```python
from build123d import *


with BuildPart() as part:
    # 草图1 → 旋转1 (revolve)
    with BuildSketch(Plane.XY, mode=Mode.PRIVATE) as revolve_1_sk:
        Polygon((10, 0), (0, 0), (0, 3.521877004), (0.272997582, 4), (0.545995165, 3.521877004), (0.818992747, 4), (1.091990329, 3.521877004), (1.364987912, 4), (1.637985494, 3.521877004), (1.910983076, 4), (2.183980659, 3.521877004), (2.456978241, 4), (2.729975823, 3.521877004), (3.002973406, 4), (3.275970988, 3.521877004), (3.548968571, 4), (3.821966153, 3.521877004), (4.094963735, 4), (4.367961318, 3.521877004), (4.6409589, 4), (4.913956482, 3.521877004), (5.186954065, 4), (5.459951647, 3.521877004), (5.732949229, 4), (6.005946812, 3.521877004), (6.278944394, 4), (6.551941976, 3.521877004), (6.824939559, 4), (7.097937141, 3.521877004), (7.236117111, 3.763882889), (10, 1), align=None)
    revolve(revolve_1_sk.sketch.rotate(Axis((10, 0, 0), (1, 0, 0)), 270), axis=Axis((10, 0, 0), (1, 0, 0)))


solid = part.part
```
The model under review builds one solid part; all positions refer to its coordinate system, in mm. Coordinates: 2 decimals unless noted, no trailing zeros. Order: outer loops, then holes, each group sorted by start corner. A loop starts at its lowest first (then second) coordinate and runs counter-clockwise, first axis right, second up. Notation, with made-up numbers: (-10, 72) -> (48, 72) arc R16 ccw to (48, 95) -> close; hole circle Ø8 at (4, 62.5). An arc over 180 degrees is marked (long way). Answer in a Markdown table with one row per item. Add a question column.
Item 1: We need section A-A on x = 8.5. Write out the cut boundary in (y, z).
Item 2: To check wall thickness, follow probe 1 along Z at (x, y) = (5.5, 1.75); probe 2 along X at (y, z) = (0, -2); probe 3 along Z at (x, y) = (7.75, -2.75). State the ranges of each line that lie inside material, in increasing order.
Item 3: We need section B-B on x = 1.5. Write out the cut boundary in (y, z), plus the area to 3 significant figures.
Final values:
| question | item | result |
|---|---|---|
| 1 | outline | circle Ø5 at (0, 0) |
| 2 | probe 1 | z = -3.14 to 3.14 |
| 2 | probe 2 | x = 0 to 9 |
| 2 | probe 3 | z = -1.73 to 1.73 |
| 3 | outline | circle Ø7.53 at (0, 0) |
| 3 | area | 44.5 mm2 |
